from build123d import *

# Parameters (mm, degrees)
SZKIC1_R                    = 4
DODANIE_WYCI_GNI_CIE1_DEPTH = 3


with BuildPart() as part:
    # Szkic1 → Dodanie-wyciągnięcie1 (new body)
    with BuildSketch(Plane(origin=(0, 0, 0), x_dir=(1, 0, 0), z_dir=(0, 1, 0))):
        with BuildLine():
            Line((-1700.695176003, -413.9172979), (-1679.663082135, -397.254434174))
            ThreePointArc((-1679.663082135, -397.254434174), (-1677.51, -389.169618943), (-1684.642632151, -384.796341157))
            Line((-1684.642632151, -384.796341157), (-1711.365640324, -387.221384291))
            ThreePointArc((-1711.365640324, -387.221384291), (-1713.508120123, -387.573596893), (-1715.577306167, -388.231428571))
            Line((-1715.577306167, -388.231428571), (-1714.649421806, -390.552857143))
            ThreePointArc((-1714.649421806, -390.552857143), (-1698.402857143, -397.520578194), (-1705.370578194, -413.767142857))
            Line((-1705.370578194, -413.767142857), (-1704.442693833, -416.088571429))
            ThreePointArc((-1704.442693833, -416.088571429), (-1702.490155803, -415.138903777), (-1700.695176003, -413.9172979))
        make_face()
        with Locations((-1684.01, -391.767695155)):
            Circle(SZKIC1_R, mode=Mode.SUBTRACT)
    extrude(amount=DODANIE_WYCI_GNI_CIE1_DEPTH)


solid = part.part
Could you check a few things on this model? Use its own coordinates, in mm. Coordinates: 2 decimals unless noted, no trailing zeros. Loops run counter-clockwise (first coordinate to the right, second up) from the corner with the lowest first, then second, coordinate; pieces in that order, holes last. Notation, with made-up numbers: (71, 57) -> (93, 57) arc R20 cw to (93, 73) -> close; hole circle Ø6 at (-8, 49). An arc over 180 degrees is marked (long way). Answer in a Markdown table with one row per item.
(1) Imagine slicing it at C-C (x = -1684.01). List the corners of the cut face in (y, z) for me.
Results found:
| item | result |
|---|---|
| outline | (0, 384.77) -> (3, 384.77) -> (3, 387.77) -> (0, 387.77) -> close; (0, 395.77) -> (3, 395.77) -> (3, 400.7) -> (0, 400.7) -> close |
(2) If I drill on probe 1 along Z at (x, y) = (-1684.01, 2.1); probe 2 along Z at (x, y) = (-1700.5, 0.2); probe 3 along X at (y, z) = (0.7, 397), over which ranges is the centre line in solid material (lowest first)?
Results found:
| item | result |
|---|---|
| probe 1 | z = 384.77 to 387.77, 395.77 to 400.7 |
| probe 2 | z = 386.24 to 394.05, 410.27 to 413.76 |
| probe 3 | x = -1698.62 to -1679.36 |
(3) Will these pins go through, and if not, where does the flat tip stop? pin 1 Ø12 at (x, z) = (-1699, 412.5) entering from -Y; pin 2 Ø1 at (y, z) = (1, 400.5) entering from -X.
Results found:
| item | result |
|---|---|
| pin 1 | stops at y = 0 |
| pin 2 | stops at x = -1697.7 |
(4) Thinking about a two-plate mould opening in Z: for faces 1 (the face through (-1713.479, 1.479, 387.567)), 2 (the face through (-1698.508, 1.479, 397.266)), 3 (the face through (-1677.464, 1.479, 389.287)), 4 (the face through (-1692, 0, 397)), which applies, released by +Z, released by -Z, zero draft, split by the parting line, or undercut?
Results found:
| item | result |
|---|---|
| face 1 | released by -Z |
| face 2 | undercut |
| face 3 | split by the parting line |
| face 4 | zero draft |
(5) Imagine slicing it at A-A (y = 0.95). List the corners of the cut face in (x, z) for me, plus the area to 3 significant figures.
Results found:
| item | result |
|---|---|
| outline | (-1715.58, 388.23) arc R15 ccw to (-1711.37, 387.22) -> (-1684.64, 384.8) arc R7 ccw to (-1679.66, 397.25) -> (-1700.7, 413.92) arc R15 ccw to (-1704.44, 416.09) -> (-1705.37, 413.77) arc R12.5 cw to (-1714.65, 390.55) -> close; hole circle Ø8 at (-1684.01, 391.77) |
| area | 423 mm^2 |
(6) Imagine slicing it at D-D (z = 402.16). List the corners of the cut face in (x, y) for me, plus the area to 3 significant figures.
Results found:
| item | result |
|---|---|
| outline | (-1697.51, 0) -> (-1685.85, 0) -> (-1685.85, 3) -> (-1697.51, 3) -> close |
| area | 35.0 mm^2 |
(7) Imagine slicing it at B-B (x = -1702). List the corners of the cut face in (y, z) for me, plus the area to 3 significant figures.
Results found:
| item | result |
|---|---|
| outline | (0, 386.37) -> (3, 386.37) -> (3, 392.56) -> (0, 392.56) -> close; (0, 411.76) -> (3, 411.76) -> (3, 414.84) -> (0, 414.84) -> close |
| area | 27.8 mm^2 |
